```python
from build123d import *

# Parameters (mm, degrees)
F1_DEPTH = 1000


with BuildPart() as f1:
    # F0 (on Front) → F1 (new body)
    with BuildSketch(Plane.XZ):
        with BuildLine():
            ThreePointArc((0, 5), (1.464466, 1.464466), (5, 0))
            Line((5, 0), (135, 0))
            ThreePointArc((135, 0), (138.535534, 1.464466), (140, 5))
            Line((140, 5), (140, 8.076507))
            ThreePointArc((140, 8.076507), (138.671049, 11.47112), (135.390639, 13.061223))
            Line((135.390639, 13.061223), (83.359361, 17.138777))
            ThreePointArc((83.359361, 17.138777), (80.078951, 18.72888), (78.75, 22.123493))
            Line((78.75, 22.123493), (78.75, 45.45))
            Line((78.75, 45.45), (84.3, 51))
            Line((84.3, 51), (84.3, 96.45))
            Line((84.3, 96.45), (78.75, 102))
            Line((78.75, 102), (61.25, 102))
            Line((61.25, 102), (55.7, 96.45))
            Line((55.7, 96.45), (55.7, 51))
            Line((55.7, 51), (61.25, 45.45))
            Line((61.25, 45.45), (61.25, 22.123493))
            ThreePointArc((61.25, 22.123493), (59.921049, 18.72888), (56.640639, 17.138777))
            Line((56.640639, 17.138777), (4.609361, 13.061223))
            ThreePointArc((4.609361, 13.061223), (1.328951, 11.47112), (0, 8.076507))
            Line((0, 8.076507), (0, 5))
        make_face()
    extrude(amount=-F1_DEPTH)


solid = f1.part
```
Part model, mm, in its own coordinate system. A direction names the side the tool comes from. Coordinates: 2 decimals unless noted, no trailing zeros. Write each loop counter-clockwise with the first axis right and the second up, starting at its lowest first coordinate (ties: lowest second). Pieces come first, ordered by that corner, then holes.
Item 1: Slice it at B-B (z = 83). Write the cut outline in (x, y), and give its area (3 significant figures).
Item 2: Mould opens along Z. For faces 1 (the face through (61.25, 493, 34)), 2 (the face through (78.75, 493, 34)), 3 (the face through (84.3, 493, 73)), 4 (the face through (69, 493, 0)) say: released by +Z, released by -Z, zero draft, split by the parting line, or undercut.
Item 3: Slice it at C-C (x = 15). Write the cut outline in (y, z), and give its area (3 significant figures).
Item 4: Pin check, flat tips, straight feed: pin 1 (7 mm diameter, centred on y = 481, z = 39, fed in from -X); pin 2 (12 mm diameter, centred on x = 24, z = 18, fed in from -Y); pin 3 (1 mm diameter, centred on y = 147.5, z = 58, fed in from +X); pin 4 (5 mm diameter, centred on x = 105.5, y = 463, fed in from +Z). Stop position of each tip, or through.
Item 5: Slice it at A-A (y = 651). Write the cut outline in (x, z), and give its area (3 significant figures).
Item 6: Which spindle directions (+Z, -Z, +X, -X, +Y, -Y) get a long thin tool onto all of the face, cutting with end or side? Do faces 5 (the face through (55.7, 493, 74)), 6 (the face through (64, 1000, 36)). Say none if no direction does.
Item 7: Probe line 1 (X direction, y = 811, z = 79); line 2 (X direction, y = 369, z = 33); line 3 (Z direction, x = 82, y = 518). List the from-to ranges inside material, lowest first.
Results found:
1. outline: (55.7, 0) - (84.3, 0) - (84.3, 1000) - (55.7, 1000) - close
1. area: 28,600 mm2
2. face 1: undercut
2. face 2: undercut
2. face 3: zero draft
2. face 4: released by -Z
3. outline: (0, 0) - (1000, 0) - (1000, 13.88) - (0, 13.88) - close
3. area: 13,900 mm2
4. pin 1: stops at x = 61.25
4. pin 2: stops at y = 0
4. pin 3: stops at x = 84.3
4. pin 4: stops at z = 15.6
5. outline: (0, 5) arc R5 ccw to (5, 0) - (135, 0) arc R5 ccw to (140, 5) - (140, 8.08) arc R5 ccw to (135.39, 13.06) - (83.36, 17.14) arc R5 cw to (78.75, 22.12) - (78.75, 45.45) - (84.3, 51) - (84.3, 96.45) - (78.75, 102) - (61.25, 102) - (55.7, 96.45) - (55.7, 51) - (61.25, 45.45) - (61.25, 22.12) arc R5 cw to (56.64, 17.14) - (4.61, 13.06) arc R5 ccw to (0, 8.08) - close
5. area: 4,190 mm2
6. face 5: +Z, -X, +Y, -Y
6. face 6: +Z, -Z, +X, -X, +Y
7. line 1: x = 55.7 to 84.3
7. line 2: x = 61.25 to 78.75
7. line 3: z = 0 to 17.44, 48.7 to 98.75
